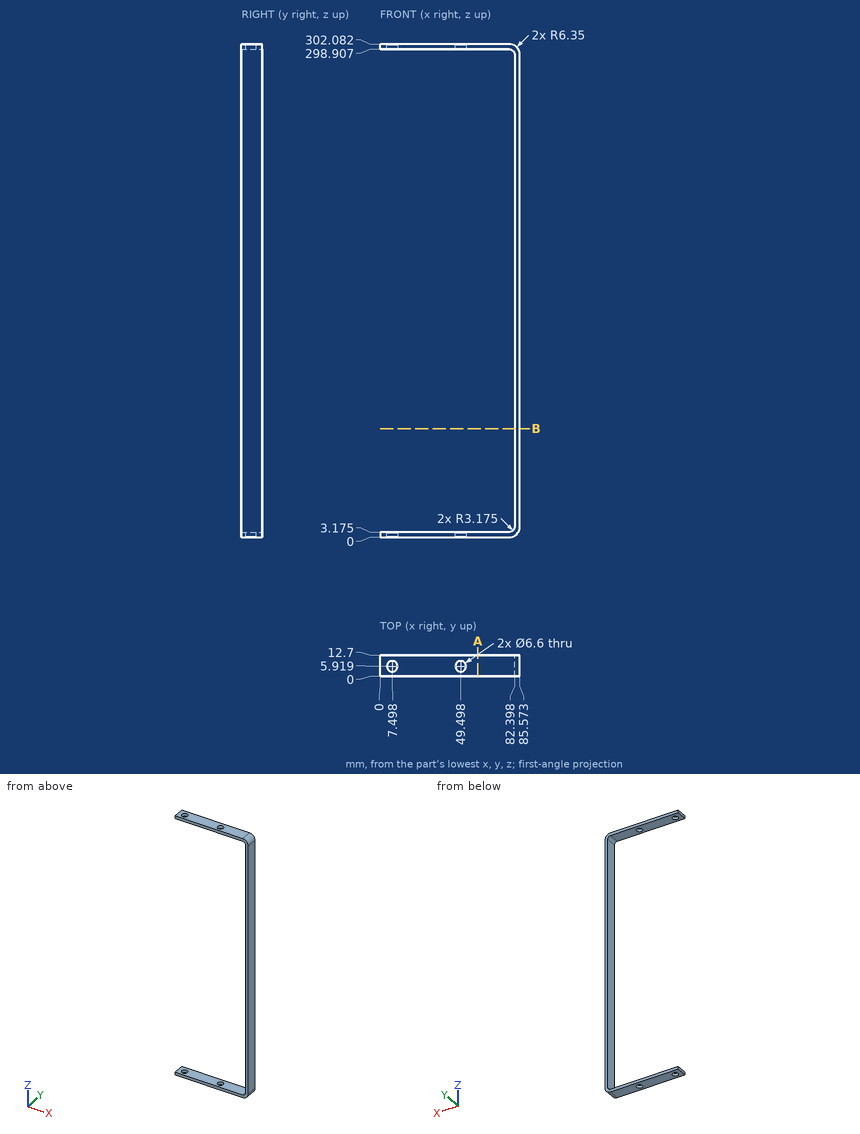
Geometry: see drawing. Coordinates: mm, zero at the bounding-box minimum. Coordinates: 2 decimals unless noted, no trailing zeros. Write each loop counter-clockwise with the first axis right and the second up, starting at its lowest first coordinate (ties: lowest second). Pieces come first, ordered by that corner, then holes. Notation, with made-up numbers: (77, -13) - (127, -13) arc R28 ccw to (127, 5) - close; hole circle Ø3 at (46.5, 21). An arc over 180 degrees is marked (long way). Put each result on its own line as item: value. Start each with the question number.
1) Ray query, L1, parallel to Z at x = 31, y = 6.25 (1 decimal); L2, parallel to X at y = 4.25, z = 46; L3, parallel to Z at x = 80, y = 8 (1 decimal). Return the intervals inside material, ascending.
2) Contact query for flat-ended pins moving along their axis: pin 1 (4 mm diameter, centred on x = 7.5, y = 5.92, fed in from -Z); pin 2 (1 mm diameter, centred on y = 2.5, z = 46, fed in from -X). Output: stop coordinate, or through.
3) Cut plane B-B (z = 66.5). Return the cut outline in (x, y), plus the area to 3 significant figures.
4) Cut plane A-A (x = 60). Return the cut outline in (y, z) (1 decimal).
Resolved:
1. L1: z = 0 to 3.2, 298.9 to 302.1
1. L2: x = 82.4 to 85.57
1. L3: z = 0 to 3.3, 298.8 to 302
2. pin 1: passes through
2. pin 2: stops at x = 82.4
3. outline: (82.4, 0) - (85.57, 0) - (85.57, 12.7) - (82.4, 12.7) - close
3. area: 40.3 mm2
4. outline: (0, 0) - (12.7, 0) - (12.7, 3.2) - (0, 3.2) - close; (0, 298.9) - (12.7, 298.9) - (12.7, 302.1) - (0, 302.1) - close
